The model under review builds one solid part; all positions refer to its coordinate system, in mm. A direction names the side the tool comes from. Give positions to 0.01 mm unless a question says otherwise; leave off trailing zeros. Order: outer loops, then holes, each group sorted by start corner. A loop starts at its lowest first (then second) coordinate and runs counter-clockwise, first axis right, second up. Notation, with made-up numbers: (45.5, 29.5) - (62.5, 29.5) arc R27 cw to (62.5, 57.5) - close; hole circle Ø4 at (39, -8.5). An arc over 180 degrees is marked (long way). Put each result on its own line as item: value.
```python
from build123d import *

# Parameters (mm, degrees)
BOSS_EXTRUDE1_DEPTH = 3
SKETCH2_W           = 6.903287468
SKETCH2_H           = 3
BOSS_EXTRUDE2_DEPTH = 60
SKETCH3_W           = 7.25
SKETCH3_H           = 3
BOSS_EXTRUDE3_DEPTH = 60
SKETCH4_W           = 2.5
SKETCH4_H           = 6.903287468
SKETCH4_H_2         = 7.25
BOSS_EXTRUDE4_DEPTH = 100


with BuildPart() as part:
    # Sketch1 → Boss-Extrude1 (new body)
    with BuildSketch(Plane(origin=(0, 0, 0), x_dir=(1, 0, 0), z_dir=(0, 1, 0))):
        with BuildLine():
            Line((10, 31), (10, 0))
            ThreePointArc((10, 0), (0, -10), (-10, 0))
            Line((-10, 0), (-10, 31))
            ThreePointArc((-10, 31), (0, 41), (10, 31))
        make_face()
        with BuildLine():
            Line((-3, 0), (-3, 31))
            ThreePointArc((-3, 31), (0, 34), (3, 31))
            Line((3, 31), (3, 0))
            ThreePointArc((3, 0), (0, -3), (-3, 0))
        make_face(mode=Mode.SUBTRACT)
    extrude(amount=BOSS_EXTRUDE1_DEPTH)

    # Sketch2 → Boss-Extrude2 (add)
    with BuildSketch(Plane(origin=(10, 0, 0), x_dir=(0, 0, -1), z_dir=(1, 0, 0))):
        with Locations((15.5, 1.5)):
            Rectangle(SKETCH2_W, SKETCH2_H)
    extrude(amount=BOSS_EXTRUDE2_DEPTH)

    # Sketch3 → Boss-Extrude3 (add)
    with BuildSketch(Plane.ZY.offset(10)):
        with Locations((-15.5, 1.5)):
            Rectangle(SKETCH3_W, SKETCH3_H)
    extrude(amount=BOSS_EXTRUDE3_DEPTH)

    # Sketch4 → Boss-Extrude4 (add)
    with BuildSketch(Plane(origin=(0, 3, 0), x_dir=(1, 0, 0), z_dir=(0, 1, 0))):
        with Locations((68.75, 15.5)):
            Rectangle(SKETCH4_W, SKETCH4_H)
        with Locations((-68.75, 15.5)):
            Rectangle(SKETCH4_W, SKETCH4_H_2)
    extrude(amount=BOSS_EXTRUDE4_DEPTH)


solid = part.part
```
(1) Wall thickness on L1, parallel to Y at x = -27.5, z = -18.5: over which ranges is the line inside the solid? List them lowest first.
The answers:
L1: 0 to 3
(2) For faces 5 (the flat face through (-5, 3, -16)), 6 (the flat face through (-69, 28, -11.875)), 7 (the flat face through (69, 28, -18.952)), 8 (the cylindrical face through (0, 1, 3)), 9 (the flat face through (10, 1, -6)), list the 3-axis set-ups (+Z, -Z, +X, -X, +Y, -Y) from which the entire face can be reached by the end or side of a thin tool; tool diameter is ignored.
The answers:
face 5: +Z, -Z, +Y
face 6: +Z, -X, +Y, -Y
face 7: -Z, +X, +Y, -Y
face 8: +Y, -Y
face 9: +Z, +X, +Y, -Y
(3) Clearance check with flat-ended pins moving along their axes: pin 1 Ø1.5 at (y, z) = (1.5, -7.5) entering from -X; pin 2 Ø0.9 at (y, z) = (2, -26.5) entering from +X. State where each tip first meets the part, or that it passes through.
The answers:
pin 1: x = -10
pin 2: x = 10
(4) Take a section at C-C, the plane x = 0. Write out the cut boundary in (y, z).
The answers:
outline: (0, -41) - (3, -41) - (3, -34) - (0, -34) - close; (0, 3) - (3, 3) - (3, 10) - (0, 10) - close
(5) The part is to be moulded in two halves that separate along Z. For faces 1 (the flat face through (-3, 1, -15)), 2 (the flat face through (10, 1, -25)), 3 (the flat face through (3, 1, -16)), 4 (the flat face through (-69, 28, -19.125)), say which applies: pulls with the +Z half, pulls with the -Z half, needs draft (parallel to the pull), parting line crosses it, or undercut.
The answers:
face 1: undercut
face 2: needs draft
face 3: undercut
face 4: pulls with the -Z half
(6) Take a section at B-B, the plane z = -17.5. Write out the cut boundary in (x, y).
The answers:
outline: (-70, 0) - (-3, 0) - (-3, 3) - (-67.5, 3) - (-67.5, 103) - (-70, 103) - close; (3, 0) - (70, 0) - (70, 103) - (67.5, 103) - (67.5, 3) - (3, 3) - close
(7) Take a section at D-D, the plane x = 45. Write out the cut boundary in (y, z), then the cut area to 3 significant figures.
The answers:
outline: (0, -18.95) - (3, -18.95) - (3, -12.05) - (0, -12.05) - close
area: 20.7 mm^2
(8) Take a section at A-A, the plane y = 90.5. Write out the cut boundary in (x, z) (3 decimals), then the cut area to 3 significant figures.
The answers:
outline: (-70, -19.125) - (-67.5, -19.125) - (-67.5, -11.875) - (-70, -11.875) - close; (67.5, -18.952) - (70, -18.952) - (70, -12.048) - (67.5, -12.048) - close
area: 35.4 mm^2
